```python
from build123d import *

# Parameters (mm, degrees)
F0_W      = 1016
F0_H      = 19.05
F1_DEPTH  = 38.1
F3_DEPTH  = 50.8
F5_DEPTH  = 76.2
F7_DEPTH  = 60.325
F9_DEPTH  = 9.525
F11_DEPTH = 60.325
F13_DEPTH = 19.05
F15_DEPTH = 9.525


with BuildPart() as f1:
    # F0 (on Front) → F1 (new body)
    with BuildSketch(Plane.XZ):
        with Locations((-508, 9.525)):
            Rectangle(F0_W, F0_H)
    extrude(amount=F1_DEPTH)

    # F2 (on face) → F3 (cut)
    with BuildSketch(Plane.XY.offset(19.05)):
        Polygon((-1016, 0), (-1016, -38.1), (-1002.3770791998, 0), align=None)
    extrude(amount=-F3_DEPTH, mode=Mode.SUBTRACT)

    # F4 (on face) → F5 (cut)
    with BuildSketch(Plane.XY.offset(19.05)):
        Polygon((-13.6229208002, 0), (0, -38.1), (0, 0), align=None)
    extrude(amount=-F5_DEPTH, mode=Mode.SUBTRACT)

    # F6 (on face) → F7 (cut)
    with BuildSketch(Plane(origin=(-888.7527181239, 317.7797346454, 0), x_dir=(-0.3366822055, -0.941618337, 0), z_dir=(-0.941618337, 0.3366822055, 0))):
        Polygon((252.7767419815, 9.525), (258.7343550339, 0), (377.9447794005, 0), (377.9447794005, 9.525), align=None)
    extrude(amount=-F7_DEPTH, mode=Mode.SUBTRACT)

    # F8 (on face) → F9 (cut)
    with BuildSketch(Plane(origin=(0, 0, 0), x_dir=(1, 0, 0), z_dir=(0, 0, -1))):
        Polygon((-951.9347650406, 38.1), (-951.9347650406, 0), (-934.7637907817, 0), align=None)
    extrude(amount=-F9_DEPTH, mode=Mode.SUBTRACT)

    # F10 (on face) → F11 (cut)
    with BuildSketch(Plane(origin=(-12.0786958733, -4.3188219751, 0), x_dir=(-0.3366822055, 0.941618337, 0), z_dir=(0.941618337, 0.3366822055, 0))):
        Polygon((-35.8756586385, 19.05), (-35.8756586385, 9.525), (45.2719508199, 9.525), (45.6329248846, 19.05), align=None)
    extrude(amount=-F11_DEPTH, mode=Mode.SUBTRACT)

    # F12 (on face) → F13 (cut)
    with BuildSketch(Plane(origin=(0, 0, 0), x_dir=(-1, 0, 0), z_dir=(0, 1, 0))):
        Polygon((524.497778814, 0), (513.499256186, 19.05), (491.502221186, 19.05), (502.500743814, 0), align=None)
    extrude(amount=-F13_DEPTH, mode=Mode.SUBTRACT)

    # F14 (on face) → F15 (cut)
    with BuildSketch(Plane.XY.offset(19.05)):
        Polygon((-64.0652349594, 0), (-81.2362092183, 0), (-64.0652349594, -38.1), align=None)
    extrude(amount=-F15_DEPTH, mode=Mode.SUBTRACT)


solid = f1.part
```
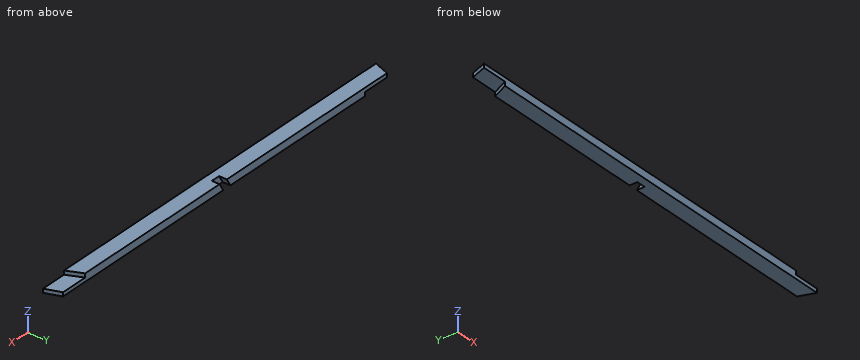
Model file for the job. Use its own axes, mm. Coordinates: 2 decimals unless noted, no trailing zeros. Write each loop counter-clockwise with the first axis right and the second up, starting at its lowest first coordinate (ties: lowest second). Pieces come first, ordered by that corner, then holes. Notation, with made-up numbers: (66, 30) - (91, 30) arc R22 cw to (91, 62) - close; hole circle Ø2 at (65, 1). An arc over 180 degrees is marked (long way). One line per question, with ' | ' between items. Start each with the question number.
Q1. Pin check, flat tips, straight feed: pin 1 (1.5 mm diameter, centred on x = -818, z = 13, fed in from +Y); pin 2 (8 mm diameter, centred on y = -6, z = 9, fed in from -X); pin 3 (10 mm diameter, centred on y = -25, z = 15, fed in from -X); pin 4 (2 mm diameter, centred on y = -29, z = 7, fed in from -X). Stop position of each tip, or through.
Q2. Cut at B-B, the plane y = -28.5. List the corners of the cut face in (x, z) (3 decimals).
Q3. Drill centre lines: line 1 (Z direction, x = -969, y = -30.5) (3 decimals); line 2 (X direction, y = -16, z = 11); line 3 (X direction, y = -11, z = 4). Where is each one in solid material? Low to high. Write a range as [from, to].
Q4. Cut at A-A, the plane z = 4.5. List the corners of the cut face in (x, y), then the cut area to 3 significant figures.
Answer below:
1) pin 1: y = 0 | pin 2: x = -1005.94 | pin 3: x = -1013.1 | pin 4: x = -948.28
2) outline: (-1012.567, 9.525) - (-947.608, 9.525) - (-947.608, 0) - (-3.433, 0) - (-3.433, 9.525) - (-68.392, 9.525) - (-68.392, 19.05) - (-1012.567, 19.05) - close
3) line 1: [9.525, 19.05] | line 2: [-1008.1, -518.15], [-496.15, -74.03] | line 3: [-939.72, -522.19], [-500.19, -9.69]
4) outline: (-951.93, -38.1) - (0, -38.1) - (-13.62, 0) - (-499.9, 0) - (-499.9, -19.05) - (-521.9, -19.05) - (-521.9, 0) - (-934.76, 0) - close | area: 35,300 mm^2
